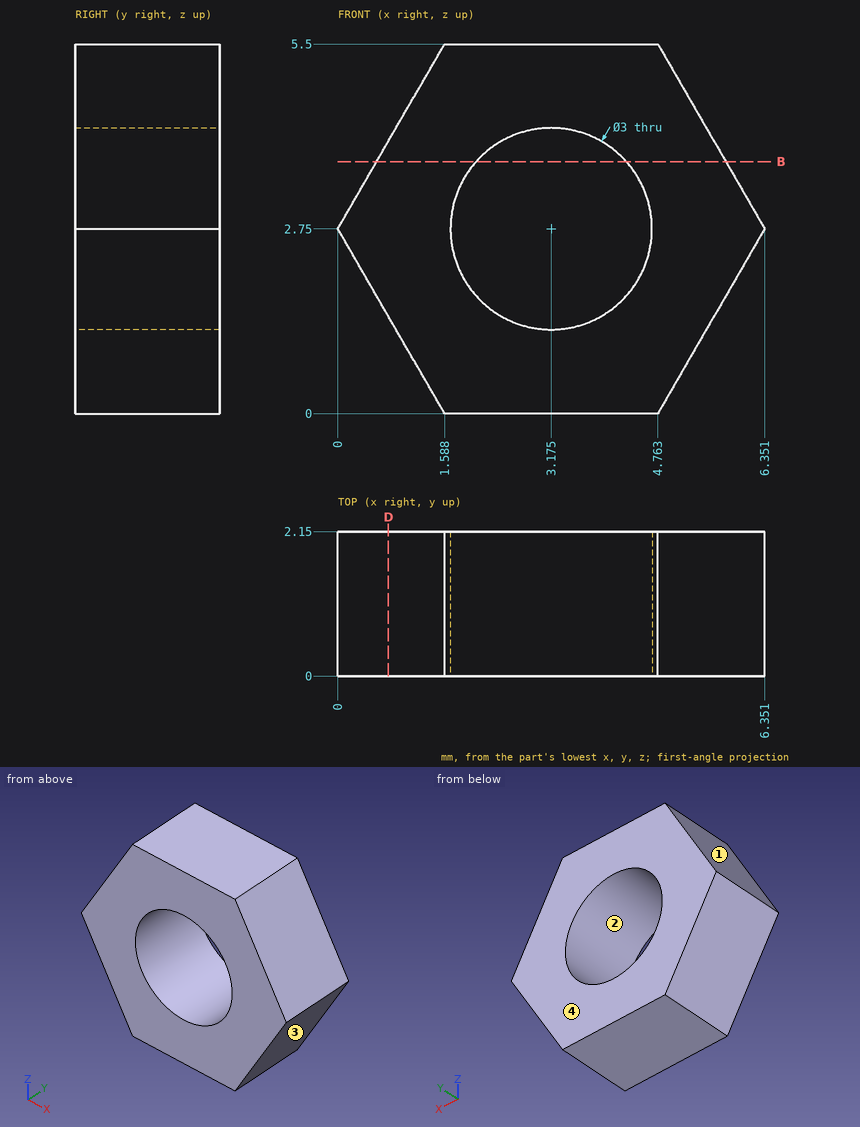
Can you work these out from the drawing? Everything is in mm from the part's minimum corner. Give positions to 0.01 mm unless a question says otherwise; leave off trailing zeros. Order: outer loops, then holes, each group sorted by start corner. A loop starts at its lowest first (then second) coordinate and runs counter-clockwise, first axis right, second up. Notation, with made-up numbers: M -33,-5.75 L 17,-5.75 A18 ccw 17,29.25 Z; hole C 44.5,57.25 d5. An arc over 180 degrees is marked long. Write item = value, one per line. Start each with the question number.
Q1. Suppose I cut it at D-D (x = 0.75). Write out the boundary of the cut face in (y, z).
Q2. We'd pull the mould along Z, two halves only. Please class the marked faces 1, 2, 3 and 4: pulls with the +Z half, pulls with the -Z half, needs draft (parallel to the pull), parting line crosses it, or undercut.
Q3. I need wall thicknesses on probe 1 along X at (y, z) = (2.05, 1.6) (1 decimal); probe 2 along Z at (x, y) = (3.5, 1.7) (1 decimal); probe 3 along Z at (x, y) = (3.75, 1.45) (1 decimal). Which ranges of each line are inside material? Lowest first, please. Write a range as [from, to].
Q4. Will this pin go through, and if not, where does the flat tip stop? pin 1 Ø1 at (y, z) = (2, 1.5) entering from -X.
Q5. Suppose I cut it at B-B (z = 3.75). Write out the boundary of the cut face in (x, y).
Check result:
q1.outline = M 0,1.45 L 2.15,1.45 L 2.15,4.05 L 0,4.05 Z
q2.face_1 = pulls with the +Z half
q2.face_2 = undercut
q2.face_3 = pulls with the -Z half
q2.face_4 = needs draft
q3.probe_1 = [0.7, 2.2], [4.1, 5.7]
q3.probe_2 = [0, 1.3], [4.2, 5.5]
q3.probe_3 = [0, 1.4], [4.1, 5.5]
q4.pin_1 = 0.43
q5.outline = M 0.58,0 L 2.06,0 L 2.06,2.15 L 0.58,2.15 Z; M 4.29,0 L 5.77,0 L 5.77,2.15 L 4.29,2.15 Z
